from build123d import *

# Parameters (mm, degrees)
SKETCH2_W               = 42.3
SKETCH2_H               = 42.3
BOSS_EXTRUDE5_DEPTH     = 39
CHAMFER4_SIZE           = 5
CUT_EXTRUDE1_START      = -8
CUT_EXTRUDE1_DEPTH      = 21
SKETCH5_R               = 20
BOSS_EXTRUDE6_DEPTH     = 4.5
SKETCH7_R               = 1.5
CUT_EXTRUDE3_DEPTH      = 4.5
SKETCH8_R               = 13.24793055
BOSS_EXTRUDE7_DEPTH     = 0.5
CUT_EXTRUDE2_DEPTH      = 53.791050378
CUT_EXTRUDE2_DEPTH_BACK = 4.5
SKETCH6_R               = 2.75


with BuildPart() as part:
    # Sketch2 → Boss-Extrude5 (new body)
    with BuildSketch(Plane.XY):
        Rectangle(SKETCH2_W, SKETCH2_H)
    extrude(amount=BOSS_EXTRUDE5_DEPTH)

    # Chamfer4
    chamfer4_edges = [part.edges().sort_by_distance(p)[0] for p in [
        (21.15, -21.15, 19.5),
        (-21.15, -21.15, 19.5),
        (-21.15, 21.15, 19.5),
        (21.15, 21.15, 19.5),
    ]]
    chamfer(chamfer4_edges, length=CHAMFER4_SIZE)

    # Sketch3 → Cut-Extrude1 (cut)
    with BuildSketch(Plane.XY.offset(39).offset(CUT_EXTRUDE1_START)):
        Polygon((-21.15, 21.15), (-21.15, 12.738640345), (-16.944320172, 16.944320172), (-12.738640345, 21.15), align=None)
        Polygon((21.15, -12.738640345), (21.15, -21.15), (12.738640345, -21.15), (16.944320172, -16.944320172), align=None)
        Polygon((12.738640345, 21.15), (21.15, 21.15), (21.15, 12.738640345), (16.944320172, 16.944320172), align=None)
        Polygon((-12.738640345, -21.15), (-21.15, -21.15), (-21.15, -12.738640345), (-16.944320172, -16.944320172), align=None)
    extrude(amount=-CUT_EXTRUDE1_DEPTH, mode=Mode.SUBTRACT)

    # Sketch5 → Boss-Extrude6 (add)
    with BuildSketch(Plane(origin=(0, 0, 0), x_dir=(-1, 0, 0), z_dir=(0, 0, -1))):
        Circle(SKETCH5_R)
    extrude(amount=BOSS_EXTRUDE6_DEPTH)

    # Sketch7 → Cut-Extrude3 (cut)
    with BuildSketch(Plane.XY.offset(39)):
        with Locations((-15.5, 15.5)):
            Circle(SKETCH7_R)
        with Locations(Location((-15.5, -15.5, 0), (0, 0, 180))):
            Circle(SKETCH7_R)
        with Locations(Location((15.5, 15.5, 0), (0, 0, 180))):
            Circle(SKETCH7_R)
        with Locations((15.5, -15.5)):
            Circle(SKETCH7_R)
    extrude(amount=-CUT_EXTRUDE3_DEPTH, mode=Mode.SUBTRACT)

    # Sketch8 → Boss-Extrude7 (add)
    with BuildSketch(Plane.XY.offset(39)):
        Circle(SKETCH8_R)
    extrude(amount=BOSS_EXTRUDE7_DEPTH)

    # Sketch6 → Cut-Extrude2 (cut, two sides: drawn at the far end of the back side and taken through both)
    with BuildSketch(Plane.XY.offset(39).offset(-CUT_EXTRUDE2_DEPTH_BACK)):
        Circle(SKETCH6_R)
    extrude(amount=CUT_EXTRUDE2_DEPTH + CUT_EXTRUDE2_DEPTH_BACK, mode=Mode.SUBTRACT)


solid = part.part
The model under review builds one solid part; all positions refer to its coordinate system, in mm. A direction names the side the tool comes from. Coordinates: 2 decimals unless noted, no trailing zeros. Loops run counter-clockwise (first coordinate to the right, second up) from the corner with the lowest first, then second, coordinate; pieces in that order, holes last.
(1) Consider section A-A, the plane z = 21. Give the boundary of the cut face in (x, y), plus the area to 3 significant figures.
Determined:
outline: (-21.15, -12.74) - (-12.74, -21.15) - (12.74, -21.15) - (21.15, -12.74) - (21.15, 12.74) - (12.74, 21.15) - (-12.74, 21.15) - (-21.15, 12.74) - close
area: 1,650 mm2
(2) Consider section C-C, the plane y = 0. Give the boundary of the cut face in (x, z).
Determined:
outline: (-21.15, 0) - (-20, 0) - (-20, -4.5) - (20, -4.5) - (20, 0) - (21.15, 0) - (21.15, 39) - (13.25, 39) - (13.25, 39.5) - (2.75, 39.5) - (2.75, 34.5) - (-2.75, 34.5) - (-2.75, 39.5) - (-13.25, 39.5) - (-13.25, 39) - (-21.15, 39) - close
(3) Insertion check: P1, Ø2.5, axis at x = 15.5, y = -15.5, coming from the +Z side; P2, Ø3.5, axis at x = -16, y = 15, coming from the +Z side; P3, Ø2.5, axis at x = -15.5, y = 15.5, coming from the -Z side. Each pin has a flat end and moves straight along its axis. Give the tip position at first contact, or say it passes through.
Determined:
P1: stops at z = 34.5
P2: stops at z = 39
P3: stops at z = 0
(4) Consider section B-B, the plane z = 36. Give the boundary of the cut face in (x, y), plus the area to 3 significant figures.
Determined:
outline: (-21.15, -16.15) - (-16.15, -21.15) - (16.15, -21.15) - (21.15, -16.15) - (21.15, 16.15) - (16.15, 21.15) - (-16.15, 21.15) - (-21.15, 16.15) - close; hole circle Ø3 at (-15.5, -15.5); hole circle Ø3 at (-15.5, 15.5); hole circle Ø5.5 at (0, 0); hole circle Ø3 at (15.5, -15.5); hole circle Ø3 at (15.5, 15.5)
area: 1,690 mm2
(5) Tool access review of faces 1 (the flat face through (18, -18, 10)), 2 (the flat face through (18, 18, 31)), 3 (the flat face through (-18, 18, 31)): name each direction out of +Z, -Z, +X, -X, +Y, -Y from which nothing blocks a thin tool from reaching the whole face with its end or side.
Determined:
face 1: +X, -Y
face 2: +X, +Y
face 3: -X, +Y
(6) Wall thickness on L1, parallel to Y at x = -15.5, z = 37.7; L2, parallel to Z at x = 19.5, y = 16.5; L3, parallel to Z at x = -13, y = 17: over which ranges is each line inside the solid? List them lowest first.
Determined:
L1: y = -21.15 to -17, -14 to 14, 17 to 21.15
L2: z = 0 to 10, 31 to 39
L3: z = 0 to 39
(7) Draft analysis for pull direction X (two halves, no side actions). For faces 4 (the flat face through (18.7, -18.6, 34.9)), 5 (the flat face through (0, 21.15, 19)), 6 (the flat face through (0, 0, 34.5)), 7 (the flat face through (-18.6, -18.7, 4.9)), state which applies: +X half, -X half, draft (parallel to the pull), parting line (faces both ways), or undercut.
Determined:
face 4: +X half
face 5: draft
face 6: undercut
face 7: -X half
